For this review, take the finished solid that the model builds, in its own axes (mm). A direction names the side the tool comes from. Coordinates: 2 decimals unless noted, no trailing zeros. Write each loop counter-clockwise with the first axis right and the second up, starting at its lowest first coordinate (ties: lowest second). Pieces come first, ordered by that corner, then holes. Notation, with made-up numbers: (-15.5, -29.75) - (23.5, -29.75) arc R24 cw to (23.5, -5.75) - close; hole circle Ø10 at (-7.5, 74). An arc over 180 degrees is marked (long way). Use one line per item in the form item = value. Start each with the question number.
1) We need section B-B (z = 0). Give the boundary of the cut face in (x, y).
2) We need section D-D (x = -2.75). Give the boundary of the cut face in (y, z), plus the area to 3 significant figures.
3) We need section C-C (y = 2.75). Give the boundary of the cut face in (x, z).
4) For L1, parallel to X at y = 1.25, z = 0; L2, parallel to Z at x = 0, y = 3; L3, parallel to X at y = 11.25, z = 0, list the stretches that pass through material, from the lowest coordinate up. Write a range as from..to.
5) Tool access review of faces 5 (the cylindrical face through (-2.579, 12.535, 1.978)), 6 (the flat face through (-2.2, 15, -0.2)): name each direction out of +Z, -Z, +X, -X, +Y, -Y from which nothing blocks a thin tool from reaching the whole face with its end or side.
6) Insertion check: P1, Ø2.5, axis at x = 1, z = 0, coming from the +Y side; P2, Ø1, axis at y = 4.5, z = 1, coming from the +X side; P3, Ø3, axis at x = 3, y = 4, coming from the +Z side. Each pin has a flat end and moves straight along its axis. Give the tip position at first contact, or say it passes through.
7) Mouldability with a two-part tool opening along Z and no side actions: class faces 1 (the flat face through (-3, 0, 0)), 2 (the cylindrical face through (2.75, 7.4, -0.09)), 3 (the flat face through (-2.05, 7, 0)), 4 (the cylindrical face through (0.867, 4.93, 3.905)) as pulls with the +Z half, pulls with the -Z half, needs draft (parallel to the pull), parting line crosses it, or undercut.
8) We need section A-A (x = 0). Give the boundary of the cut face in (y, z).
Autodesk Inventor part; units mm, degrees
ref_plane "YZ Plane" through (0, 0, 0) normal (1, 0, 0) x (0, 1, 0)
ref_plane "XZ Plane" through (0, 0, 0) normal (0, 1, 0) x (-1, 0, 0)
ref_plane "XY Plane" through (0, 0, 0) normal (0, 0, 1) x (1, 0, 0)
sketch "Sketch1" plane through (0, 0, 0) normal (0, 1, 0) x (-1, 0, 0)
  arc A0 (2.05, 1.833) -> (2.05, -1.833) centre (0, 0) ccw
  line L0 (-2.75, 2.2253) -> (-2.75, -2.0609)
  circle A1 centre (0, 0) radius 4
  line L1 (2.05, 1.833) -> (2.05, -1.833)
  dimension "d0" = 5.5
  dimension "d3" = 8
  dimension "d4" = 4.8
extrude "Extrusion1" add sketch "Sketch1" along normal blind 15
sketch "Sketch2" plane through (0, 15, 0) normal (0, 1, 0) x (1, 0, 0)
  circle A0 centre (0, 0) radius 3.25
  circle A1 centre (0, 0) radius 4
  dimension "d7" = 6.5
extrude "Extrusion2" cut sketch "Sketch2" against normal blind 5
properties part number "5.5x4.8"
Determined:
q1.outline = (-4, 0) - (-2.05, 0) - (-2.05, 15) - (-3.25, 15) - (-3.25, 10) - (-4, 10) - close; (2.75, 0) - (4, 0) - (4, 10) - (3.25, 10) - (3.25, 15) - (2.75, 15) - close
q2.outline = (0, -2.9) - (10, -2.9) - (10, -1.73) - (15, -1.73) - (15, 1.73) - (10, 1.73) - (10, 2.9) - (0, 2.9) - close
q2.area = 75.4 mm²
q3.outline = circle Ø8 at (0, 0); hole (-2.05, -1.83) arc R2.75 ccw (long way) to (-2.05, 1.83) - close
q4.L1 = -4..-2.05, 2.75..4
q4.L2 = -4..-2.75, 2.75..4
q4.L3 = -3.25..-2.05, 2.75..3.25
q5.face_5 = +Y
q5.face_6 = +Z, -Z, +X, -X, +Y
q6.P1 = through
q6.P2 = 3.97
q6.P3 = 3.71
q7.face_1 = needs draft
q7.face_2 = undercut
q7.face_3 = undercut
q7.face_4 = parting line crosses it
q8.outline = (0, -4) - (10, -4) - (10, -3.25) - (15, -3.25) - (15, -2.75) - (0, -2.75) - close; (0, 2.75) - (15, 2.75) - (15, 3.25) - (10, 3.25) - (10, 4) - (0, 4) - close
